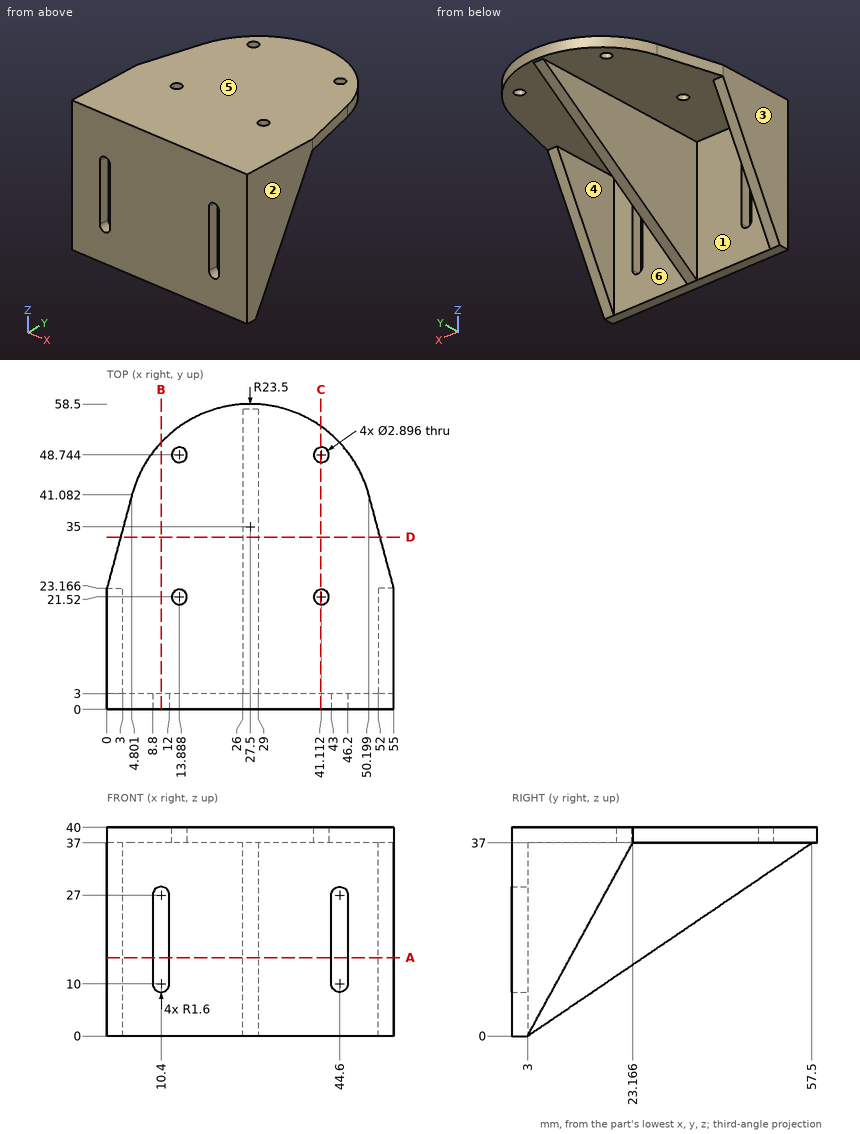
Can you work these out from the drawing? Everything is in mm from the part's minimum corner. A direction names the side the tool comes from. Round coordinates to 2 decimals unless told otherwise and drop trailing zeros. Write each loop counter-clockwise with the first axis right and the second up, starting at its lowest first coordinate (ties: lowest second). Pieces come first, ordered by that corner, then holes. Notation, with made-up numbers: M 88.25,-18 L 141.25,-18 A23 ccw 141.25,12 Z; hole C 42,68.5 d3. An arc over 180 degrees is marked long. Use a Markdown table: item, result.
Item 1: For pin 1 Ø18.5 at (x, z) = (45, 24) entering from +Y (1 decimal); pin 2 Ø6 at (y, z) = (48, 35.5) entering from -X; pin 3 Ø22 at (y, z) = (18, 15) entering from +X; pin 4 Ø18.5 at (y, z) = (36, 22.5) entering from +X, each with a flat end and sliding along its axis, tell me the tip position at first contact or that it passes through.
Found:
| item | result |
|---|---|
| pin 1 | stops at y = 19.4 |
| pin 2 | stops at x = 6.43 |
| pin 3 | stops at x = 55 |
| pin 4 | stops at x = 29 |
Item 2: We'd pull the mould along X, two halves only. Please class the marked faces 1, 2, 3 and 4: released by +X, released by -X, zero draft, split by the parting line, or undercut.
Found:
| item | result |
|---|---|
| face 1 | undercut |
| face 2 | released by +X |
| face 3 | released by -X |
| face 4 | undercut |
Item 3: I want a section at A-A (z = 15). List the corners of the cut face in (x, y) for me (1 decimal).
Found:
| item | result |
|---|---|
| outline | M 0,0 L 8.8,0 L 8.8,3 L 3,3 L 3,11.2 L 0,11.2 Z; M 12,0 L 43,0 L 43,3 L 29,3 L 29,25.1 L 26,25.1 L 26,3 L 12,3 Z; M 46.2,0 L 55,0 L 55,11.2 L 52,11.2 L 52,3 L 46.2,3 Z |
Item 4: I want a section at B-B (x = 10.4). List the corners of the cut face in (y, z) for me, and give its area (3 significant figures).
Found:
| item | result |
|---|---|
| outline | M 0,0 L 3,0 L 3,8.4 L 0,8.4 Z; M 0,28.6 L 3,28.6 L 3,37 L 51.12,37 L 51.12,40 L 0,40 Z |
| area | 204 mm2 |
Item 5: If I drill on line 1 along Z through (x, y) = (23, 6); line 2 along Y through (x, z) = (6, 2); line 3 along X through (y, z) = (28, 34.5), over which ranges is the centre line in solid material (lowest first)? Write a range as [from, to].
Found:
| item | result |
|---|---|
| line 1 | z = [37, 40] |
| line 2 | y = [0, 3] |
| line 3 | x = [26, 29] |
Item 6: I want a section at D-D (y = 33). List the corners of the cut face in (x, z) for me (1 decimal).
Found:
| item | result |
|---|---|
| outline | M 2.6,37 L 26,37 L 26,20.4 L 29,20.4 L 29,37 L 52.4,37 L 52.4,40 L 2.6,40 Z |
Item 7: Which directions (+Z, -Z, +X, -X, +Y, -Y) give clear straight access to the entire face, cutting with the end or side of a thin tool? Please do the marked faces 5 and 6.
Found:
| item | result |
|---|---|
| face 5 | +Z, +X, -X, +Y, -Y |
| face 6 | -Z, +Y |
Item 8: I want a section at C-C (x = 41). List the corners of the cut face in (y, z) for me (1 decimal).
Found:
| item | result |
|---|---|
| outline | M 0,0 L 3,0 L 3,37 L 20.1,37 L 20.1,40 L 0,40 Z; M 23,37 L 47.3,37 L 47.3,40 L 23,40 Z; M 50.2,37 L 54.2,37 L 54.2,40 L 50.2,40 Z |
